```python
from build123d import *

# Parameters (mm, degrees)
ESQUISSE1_R        = 1.05
BOSS_EXTRU_1_DEPTH = 1.53


with BuildPart() as part:
    # Esquisse1 → Boss.-Extru.1 (new body)
    with BuildSketch(Plane.XY):
        with BuildLine():
            Line((10.206015929, 5), (10.206015929, 40))
            ThreePointArc((10.206015929, 40), (7.206015929, 43), (4.206015929, 40))
            Line((4.206015929, 40), (4.206015929, 5))
            Line((4.206015929, 5), (2.371015929, 0))
            Line((2.371015929, 0), (0.706015929, 0))
            Line((0.706015929, 0), (-0.958984071, 0))
            Line((-0.958984071, 0), (-2.793984071, 5))
            Line((-2.793984071, 5), (-2.793984071, 48.5))
            ThreePointArc((-2.793984071, 48.5), (-4.343984071, 50.05), (-2.793984071, 51.6))
            Line((-2.793984071, 51.6), (-2.793984071, 60))
            Line((-2.793984071, 60), (17.206015929, 60))
            Line((17.206015929, 60), (17.206015929, 51.6))
            ThreePointArc((17.206015929, 51.6), (18.756015929, 50.05), (17.206015929, 48.5))
            Line((17.206015929, 48.5), (17.206015929, 5))
            Line((17.206015929, 5), (15.371015929, 0))
            Line((15.371015929, 0), (13.706015929, 0))
            Line((13.706015929, 0), (12.041015929, 0))
            Line((12.041015929, 0), (10.206015929, 5))
        make_face()
        with Locations((17.206015929, 50.05)):
            Circle(ESQUISSE1_R, mode=Mode.SUBTRACT)
        with Locations((-2.793984071, 50.05)):
            Circle(ESQUISSE1_R, mode=Mode.SUBTRACT)
    extrude(amount=BOSS_EXTRU_1_DEPTH)


solid = part.part
```
Can you work these out from the model? Positions are in its coordinate system, mm. A direction names the side the tool comes from. Coordinates: 2 decimals unless noted, no trailing zeros. Write each loop counter-clockwise with the first axis right and the second up, starting at its lowest first coordinate (ties: lowest second). Pieces come first, ordered by that corner, then holes. Notation, with made-up numbers: M -22.75,2.5 L 29.25,2.5 A16 ccw 29.25,26.5 Z; hole C 11,-22 d5. An arc over 180 degrees is marked long. Answer as CSV lines item,"result".
Item 1: On a 3-axis mill with a long thin cutter (end or side, diameter ignored), from which of +Z, -Z, +X, -X, +Y, -Y can I reach the whole of each face in a straight line? I mean faces 5 (the flat face through (17.206, 56, 1)), 6 (the flat face through (17.206, 27, 1)), 7 (the flat face through (-2.794, 26, 1)), 8 (the flat face through (10.206, 22, 1)), 9 (the flat face through (-2.794, 56, 1)). Say none if no direction works.
Geometry results:
face 5,"+Z, -Z, +X, +Y"
face 6,"+Z, -Z, +X, -Y"
face 7,"+Z, -Z, -X, -Y"
face 8,"+Z, -Z, -Y"
face 9,"+Z, -Z, -X, +Y"
Item 2: I'm going to push flat-ended pins straight in: P1, Ø0.8, axis at y = 26, z = 1, coming from the +X side; P2, Ø0.5, axis at y = 25, z = 1, coming from the -X side; P3, Ø8, axis at x = 13, y = 49.5, coming from the -Z side. Where does each tip first touch, or does it pass through?
Geometry results:
P1,"stops at x = 17.21"
P2,"stops at x = -2.79"
P3,"stops at z = 0"
Item 3: We'd pull the mould along Y, two halves only. Please class faces 1 (the flat face through (16.3, 2.53, 0.75)), 2 (the flat face through (7, 60, 1)), 3 (the flat face through (2, 37, 0)), 4 (the cylindrical face through (17.07, 51.09, 0.75)): +Y half, -Y half, draft (parallel to the pull), parting line (faces both ways), or undercut.
Geometry results:
face 1,"-Y half"
face 2,"+Y half"
face 3,"draft"
face 4,"undercut"
Item 4: Imagine slicing it at C-C on y = 12. List the corners of the cut face in (x, z) for me, plus the area to 3 significant figures.
Geometry results:
outline,"M -2.79,0 L 4.21,0 L 4.21,1.53 L -2.79,1.53 Z; M 10.21,0 L 17.21,0 L 17.21,1.53 L 10.21,1.53 Z"
area,"21.4 mm2"
Item 5: Imagine slicing it at B-B on z = 0.3. List the corners of the cut face in (x, y) for me.
Geometry results:
outline,"M -2.79,5 L -0.96,0 L 2.37,0 L 4.21,5 L 4.21,40 A3 cw 10.21,40 L 10.21,5 L 12.04,0 L 15.37,0 L 17.21,5 L 17.21,48.5 A1.55 ccw 17.21,51.6 L 17.21,60 L -2.79,60 L -2.79,51.6 A1.55 ccw -2.79,48.5 Z; hole C -2.79,50.05 d2.1; hole C 17.21,50.05 d2.1"
Item 6: Please list where these lines run through material, in increasing order: line 1 along X through (y, z) = (36, 1.05); line 2 along Y through (x, z) = (17.25, 0.9); line 3 along X through (y, z) = (55.5, 0.7).
Geometry results:
line 1,"x = -2.79 to 4.21, 10.21 to 17.21"
line 2,"y = 48.5 to 49, 51.1 to 51.6"
line 3,"x = -2.79 to 17.21"
Item 7: Imagine slicing it at D-D on x = 5.5. List the corners of the cut face in (y, z) for me.
Geometry results:
outline,"M 42.47,0 L 60,0 L 60,1.53 L 42.47,1.53 Z"
Item 8: Imagine slicing it at A-A on y = 50.05. List the corners of the cut face in (x, z) for me.
Geometry results:
outline,"M -4.34,0 L -3.84,0 L -3.84,1.53 L -4.34,1.53 Z; M -1.74,0 L 16.16,0 L 16.16,1.53 L -1.74,1.53 Z; M 18.26,0 L 18.76,0 L 18.76,1.53 L 18.26,1.53 Z"
